The listing builds one solid part. Answer for the finished solid, in the listing's coordinates (mm). Face numbers are marked on the shaded views. Give positions to 0.01 mm unless a question says otherwise; leave off trailing zeros. Loops run counter-clockwise (first coordinate to the right, second up) from the corner with the lowest first, then second, coordinate; pieces in that order, holes last. Notation, with made-up numbers: (29.5, 78) - (52.5, 78) arc R18 ccw to (52.5, 88) - close; hole circle Ø8 at (-39, 8.25). An arc over 180 degrees is marked (long way). Answer as CSV lines item,"result". Start each with the question number.
1) A cutting plane is placed at B-B (z = 1). Give the number of separate pieces and of enclosed holes in the cut face, and give its area (3 significant figures).
2) A cutting plane is placed at C-C (y = 0). Determine the outline of the cut face in (x, z).
3) A cutting plane is placed at A-A (y = -10). Determine the outline of the cut face in (x, z), and give its area (3 significant figures).
4) For a pull along X with two mould halves and no side action, classify the marked faces 1, 2, 3 and 4 as pulls with the +X half, pulls with the -X half, needs draft (parallel to the pull), parting line crosses it, or undercut.
5) Find the intervals of material crossed by line 1 along X through (y, z) = (-13, 1.5); line 2 along Y through (x, z) = (-35.25, 3.5); line 3 along Y through (x, z) = (12.75, 5), in increasing order.
Autodesk Inventor part; units mm, degrees
ref_plane "YZ Plane" through (0, 0, 0) normal (1, 0, 0) x (0, 1, 0)
ref_plane "XZ Plane" through (0, 0, 0) normal (0, 1, 0) x (-1, 0, 0)
ref_plane "XY Plane" through (0, 0, 0) normal (0, 0, 1) x (1, 0, 0)
sketch "Sketch1" plane through (0, 0, 0) normal (0, 0, 1) x (1, 0, 0)
  line L0 (-43.75, 33) -> (43.75, 33)
  line L1 (43.75, 33) -> (43.75, -33)
  line L2 (43.75, -33) -> (-43.75, -33)
  line L3 (-43.75, -33) -> (-43.75, 33)
  point P0 (0, 0)
  point P1 (0, 33)
  point P2 (-43.75, 0)
  dimension "d0" = 87.5
  dimension "d1" = 66
extrude "Extrusion1" add sketch "Sketch1" along normal blind 8
sketch "Sketch4" plane through (0, 0, 8) normal (0, 0, 1) x (1, 0, 0)
  line L0 (43.75, 33) -> (-43.75, 33)
  line L1 (-43.75, 33) -> (-43.75, -33)
  circle A0 centre (-35.25, 24) radius 5
  circle A1 centre (-35.25, -24) radius 5
  line L2 (-43.75, -33) -> (43.75, -33)
  point P0 (0, 0)
  dimension "d27" = 8.5
  dimension "d28" = 9
  dimension "d29" = 10
  dimension "d30" = 9
extrude "Extrusion4" cut sketch "Sketch4" against normal through all
sketch "Sketch5" plane through (0, 0, 8) normal (0, 0, 1) x (1, 0, 0)
  circle A0 centre (-23.0012, 0) radius 4
  circle A1 centre (-23.0012, 0) radius 7.5
  line L0 (-43.75, 33) -> (-43.75, -33)
  line L1 (43.75, 33) -> (-43.75, 33)
  circle A2 centre (-23.0012, 0) radius 7
  point P0 (0, 0)
  point P1 (-43.75, 0)
  dimension "d24" = 15
  dimension "d33" = 20.7488
extrude "Extrusion5" cut sketch "Sketch5" against normal through all contours A0 | A1 | A2
sketch "Sketch6" plane through (0, 0, 8) normal (0, 0, 1) x (1, 0, 0)
  circle A0 centre (-33.7512, 10) radius 1.75
  circle A1 centre (-12.2512, 10) radius 1.75
  circle A2 centre (-12.2512, -10) radius 1.75
  circle A3 centre (-33.7512, -10) radius 1.75
  line L0 (-33.7512, 10) -> (-12.2512, 10)
  line L1 (-12.2512, 10) -> (-12.2512, -10)
  line L2 (-12.2512, -10) -> (-33.7512, -10)
  line L3 (-33.7512, -10) -> (-33.7512, 10)
  line L4 (-33.7512, 10) -> (-12.2512, -10) construction
  line L5 (-12.2512, 10) -> (-33.7512, -10) construction
  circle A4 centre (-23.0012, 0) radius 7.5
  line L6 (-43.75, 33) -> (-43.75, -33)
  point P0 (0, 0)
  point P1 (-23.0012, 0)
  dimension "d35" = 3.5
  dimension "d36" = 21.5
  dimension "d37" = 20
extrude "Extrusion6" cut sketch "Sketch6" against normal through all contours L0 L3 A0 | A0 L3 L0 | L0 L1 A1 | A1 L1 L0 | L3 L2 A3 | A3 L2 L3 | L1 L2 A2 | A2 L2 L1
sketch "Sketch7" plane through (0, 0, 8) normal (0, 0, 1) x (1, 0, 0)
  point P0 (0, 0)
sketch "Sketch8" plane through (0, 0, 0) normal (0, 0, -1) x (-1, 0, 0)
  line L0 (-35.75, -33) -> (-43.75, -33)
  line L1 (-43.75, -33) -> (-43.75, 33)
  line L2 (-43.75, 33) -> (-35.75, 33)
  line L3 (-35.75, 33) -> (-35.75, -33)
  line L4 (-8.75, -33) -> (-16.75, -33)
  line L5 (-16.75, -33) -> (-16.75, 33)
  line L6 (-16.75, 33) -> (-8.75, 33)
  line L7 (-8.75, 33) -> (-8.75, -33)
  line L8 (-44.55, -20.5) -> (-44.55, -29.5)
  point P0 (0, 0)
  point P1 (-39.75, -28)
  point P2 (-39.75, -13)
  point P3 (-39.75, 13)
  point P4 (-39.75, 28)
  dimension "d38" = 4
  dimension "d39" = 5
  dimension "d40" = 15
  dimension "d41" = 5
  dimension "d42" = 15
  dimension "d56" = 26
hole "Hole1" at (39.75, 28, 0) direction (0, 0, 1) diameter 3.5 end through all
move faces "Move1" translate (2, 0, 0) faces at (43.75, -11, 2.6667)
pattern_linear "Rectangular Pattern2" count 2 spacing 15 along (0, -1, 0) count 2 spacing 41 along (0, -1, 0) of "Hole1"
pattern_linear "Rectangular Pattern3" count 2 spacing 27 along (-1, 0, 0) of "Hole1", "Rectangular Pattern2"
sketch "Sketch10" plane through (-43.75, 33, 8) normal (0, 1, 0) x (1, 0, 0)
  line L0 (0, 8) -> (0, 0)
  point P0 (43.75, 8)
  point P1 (8.5, 4)
  point P2 (0, 4)
  dimension "d66" = 8.5
hole "Hole2" at (-35.25, 33, 4) direction (0, -1, 0) diameter 4.134 depth 7.45 tip angle 118
sketch "Sketch11" plane through (-43.75, -33, 0) normal (0, -1, 0) x (1, 0, 0)
  line L0 (0, 0) -> (0, 8)
  point P0 (43.75, 0)
  point P1 (8.5, 4)
  point P2 (0, 4)
  dimension "d74" = 8.5
hole "Hole3" at (-35.25, -33, 4) direction (0, 1, 0) diameter 4.134 depth 7.45 tip angle 118
equation "\"d30\" = d28"
properties part number "0005-10-011" material "Wood (Maple)"
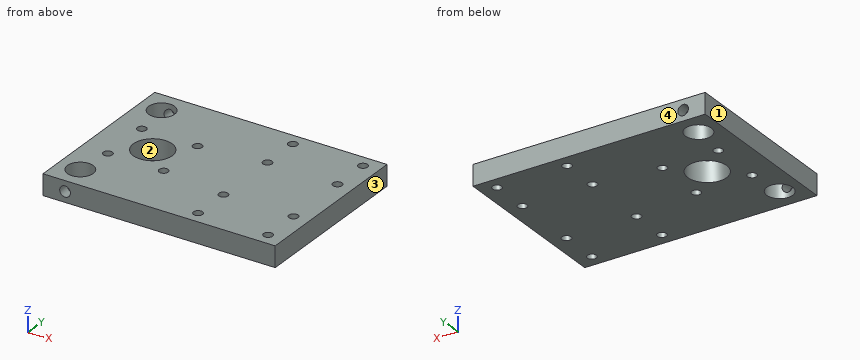
Ans:
1,separate pieces,"1"
1,enclosed holes,"15"
1,area,"5,460 mm2"
2,outline,"(-43.75, 0) - (-30.5, 0) - (-30.5, 8) - (-43.75, 8) - close; (-15.5, 0) - (45.75, 0) - (45.75, 8) - (-15.5, 8) - close"
3,outline,"(-43.75, 0) - (-35.5, 0) - (-35.5, 8) - (-43.75, 8) - close; (-32, 0) - (-14, 0) - (-14, 8) - (-32, 8) - close; (-10.5, 0) - (45.75, 0) - (45.75, 8) - (-10.5, 8) - close"
3,area,"660 mm2"
4,face 1,"pulls with the -X half"
4,face 2,"undercut"
4,face 3,"pulls with the +X half"
4,face 4,"needs draft"
5,line 1,"-43.75 to 11, 14.5 to 38, 41.5 to 45.75"
5,line 2,"-19 to -10.9, -9.1 to 9.1, 10.9 to 19"
5,line 3,"-33 to -29.75, -26.25 to -14.75, -11.25 to 11.25, 14.75 to 26.25, 29.75 to 33"
